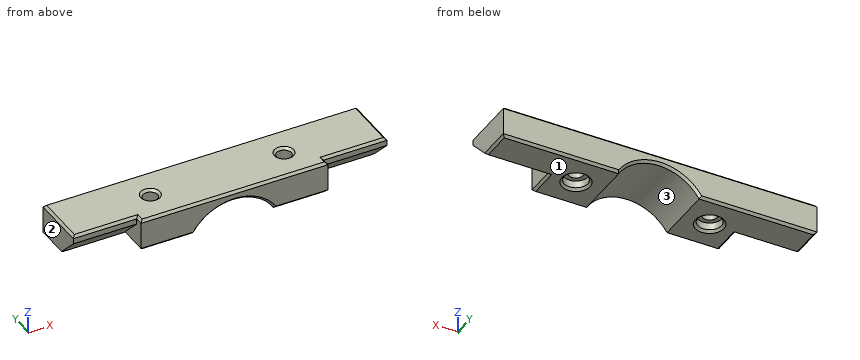
from build123d import *

# Parameters (mm, degrees)
SKIZZE1_W                       = 59
SKIZZE1_H                       = 20
AUFSATZ_LINEAR_AUSTRAGEN1_DEPTH = 10
AUFSATZ_LINEAR_AUSTRAGEN2_DEPTH = 20
SKIZZE3_R                       = 15
SCHNITT_LINEAR_AUSTRAGEN1_DEPTH = 20
SKIZZE4_R                       = 2.3
SCHNITT_LINEAR_AUSTRAGEN2_DEPTH = 20
SKIZZE5_R                       = 3.75
SCHNITT_LINEAR_AUSTRAGEN3_DEPTH = 3
SCHNITT_LINEAR_AUSTRAGEN4_DEPTH = 20
FASE3_SIZE                      = 0.75


with BuildPart() as part:
    # Skizze1 → Aufsatz-Linear austragen1 (new body)
    with BuildSketch(Plane.XY):
        with Locations((0, 10)):
            Rectangle(SKIZZE1_W, SKIZZE1_H)
    extrude(amount=AUFSATZ_LINEAR_AUSTRAGEN1_DEPTH)

    # Skizze2 → Aufsatz-Linear austragen2 (add)
    with BuildSketch(Plane.ZY.offset(29.5)):
        Polygon((10, 0), (0, 10), (0, 20), (10, 20), align=None)
    aufsatz_linear_austragen2 = extrude(amount=AUFSATZ_LINEAR_AUSTRAGEN2_DEPTH)

    # Spiegeln1: Aufsatz-Linear austragen2 across plane
    add(aufsatz_linear_austragen2.mirror(Plane(origin=(0, 0, 0), x_dir=(0, 0, 1), z_dir=(1, 0, 0))))

    # Skizze3 → Schnitt-Linear austragen1 (cut)
    with BuildSketch(Plane.XZ):
        with Locations((0, -8)):
            Circle(SKIZZE3_R)
    extrude(amount=-SCHNITT_LINEAR_AUSTRAGEN1_DEPTH, mode=Mode.SUBTRACT)

    # Skizze4 → Schnitt-Linear austragen2 (cut)
    with BuildSketch(Plane(origin=(0, 0, 0), x_dir=(-1, 0, 0), z_dir=(0, 0, -1))):
        with Locations((-21.09428877, 10)):
            Circle(SKIZZE4_R)
        with Locations(Location((21.09428877, 10, 0), (0, 0, 180))):
            Circle(SKIZZE4_R)
    extrude(amount=-SCHNITT_LINEAR_AUSTRAGEN2_DEPTH, mode=Mode.SUBTRACT)

    # Skizze5 → Schnitt-Linear austragen3 (cut)
    with BuildSketch(Plane(origin=(0, 0, 0), x_dir=(-1, 0, 0), z_dir=(0, 0, -1))):
        with Locations((-21.09428877, 10)):
            Circle(SKIZZE5_R)
        with Locations((21.09428877, 10)):
            Circle(SKIZZE5_R)
    extrude(amount=-SCHNITT_LINEAR_AUSTRAGEN3_DEPTH, mode=Mode.SUBTRACT)

    # Skizze6 → Schnitt-Linear austragen4 (cut)
    with BuildSketch(Plane.ZY.offset(49.5)):
        Polygon((10, 2.5), (4.852604626, 2.5), (4.852604626, -2.668604054), (13.586779437, -2.788104879), (13.586779437, 2.151024835), align=None)
    schnitt_linear_austragen4 = extrude(amount=-SCHNITT_LINEAR_AUSTRAGEN4_DEPTH, mode=Mode.SUBTRACT)

    # Spiegeln3: Schnitt-Linear austragen4 across plane
    add(schnitt_linear_austragen4.mirror(Plane(origin=(0, 0, 0), x_dir=(0, 0, 1), z_dir=(1, 0, 0))), mode=Mode.SUBTRACT)

    # Fase3
    fase3_edges = [part.edges().sort_by_distance(p)[0] for p in [
        (39.5, 2.5, 10),
        (29.5, 1.25, 10),
        (0, 0, 10),
        (-29.5, 5, 0),
        (-49.5, 15, 0),
        (49.5, 15, 0),
        (-31.09428877, 20, 0),
        (21.09428877, 0, 0),
        (0, 20, 7),
        (0, 0, 7),
        (0, 20, 10),
        (29.5, 5, 0),
        (23.39428877, 10, 10),
        (-21.09428877, 0, 0),
        (-23.39428877, 10, 10),
        (31.09428877, 20, 0),
        (24.84428877, 10, 0),
        (-17.34428877, 10, 0),
        (-49.5, 11.25, 10),
        (-39.5, 2.5, 10),
        (-29.5, 1.25, 10),
        (49.5, 11.25, 10),
    ]]
    chamfer(fase3_edges, length=FASE3_SIZE)


solid = part.part
Can you work these out from the model? Positions are in its coordinate system, mm. Face numbers are marked on the shaded views. Give positions to 0.01 mm unless a question says otherwise; leave off trailing zeros. Order: outer loops, then holes, each group sorted by start corner. A loop starts at its lowest first (then second) coordinate and runs counter-clockwise, first axis right, second up. Notation, with made-up numbers: M 52,-0.5 L 83,-0.5 A18 cw 83,7.5 Z; hole C 75,87 d6. An arc over 180 degrees is marked long. Use a Markdown table: item, result. Add a question column.
Item 1: Suppose I cut it at A-A (x = -30.5). List the corners of the cut face in (y, z) for me.
Item 2: If I drill on L1, parallel to Y at x = 22.5, z = 2; L2, parallel to X at y = 18.75, z = 5.25; L3, parallel to Z at x = -43.5, y = 4.5, over which ranges is the centre line in solid material (lowest first)? Write a range as [from, to].
Item 3: We'd pull the mould along X, two halves only. Please class the marked faces 1, 2 and 3: +X half, -X half, draft (parallel to the pull), parting line (faces both ways), or undercut.
Item 4: Will these pins go through, and if not, where does the flat tip stop? pin 1 (5.5 mm diameter, centred on x = -21.09, y = 10, fed in from +Z); pin 2 (2 mm diameter, centred on x = 33, y = 4.5, fed in from -Z); pin 3 (8.5 mm diameter, centred on x = 21.09, y = 10, fed in from -Z).
Answer sheet:
| question | item | result |
|---|---|---|
| 1 | outline | M 2.5,7.5 L 10,0 L 19.25,0 L 20,0.75 L 20,9.25 L 19.25,10 L 3.25,10 L 2.5,9.25 Z |
| 2 | L1 | y = [0, 6.52], [13.48, 20] |
| 2 | L2 | x = [-49.5, -7.03], [7.03, 49.5] |
| 2 | L3 | z = [5.5, 10] |
| 3 | face 1 | draft |
| 3 | face 2 | -X half |
| 3 | face 3 | undercut |
| 4 | pin 1 | stops at z = 9.7 |
| 4 | pin 2 | stops at z = 4.5 |
| 4 | pin 3 | stops at z = 0.25 |
